The listing builds one solid part. Answer for the finished solid, in the listing's coordinates (mm). Face numbers are marked on the shaded views. A direction names the side the tool comes from. Round coordinates to 2 decimals unless told otherwise and drop trailing zeros. Loops run counter-clockwise (first coordinate to the right, second up) from the corner with the lowest first, then second, coordinate; pieces in that order, holes last. Notation, with made-up numbers: M 1,-13 L 43,-13 A36 cw 43,26 Z; hole C 39.5,35.25 d2. An arc over 180 degrees is marked long. Put each result on its own line as item: value. Start each with the question number.
(1) Section A-A, the plane x = 18.5 is taken. Determine the outline of the cut face in (y, z), then the cut area to 3 significant figures.
(2) Determine the mould class of the marked faces 6, 7 and 8 for opening direction Y: released by +Y, released by -Y, zero draft, split by the parting line, or undercut.
(3) Section C-C, the plane y = -60 is taken. Determine the outline of the cut face in (x, z), then the cut area to 3 significant figures.
(4) Section D-D, the plane y = 11 is taken. Determine the outline of the cut face in (x, z).
(5) Flat-ended cylindrical pins translate along their axes: P1, Ø22, axis at y = -7, z = 12, coming from the -X side; P2, Ø6, axis at y = -37, z = 26.5, coming from the -X side; P3, Ø2, axis at x = 184.5, z = 16.5, coming from the +Y side; P4, Ø12, axis at x = 85.5, y = -54, coming from the +Z side. Find the tip coordinate at first contact, or state that the pin passes through.
(6) Which of the six approach directions +Z, -Z, +X, -X, +Y, -Y give full straight-line access (tool end or side, diameter ignored) to the marked faces 1, 2, 3, 4 and 5?
(7) Straight lines are drawn through the part: line 1 (Y direction, x = 148, z = 12); line 2 (X direction, y = 34.5, z = 11); line 3 (Y direction, x = 180.5, z = 21). For each, find the intervals that lie inside material, in ascending order.
(8) Section B-B, the plane y = 36.5 is taken. Determine the outline of the cut face in (x, z), then the cut area to 3 significant figures.
```python
from build123d import *

# Parameters (mm, degrees)
BOSS_EXTRU_1_DEPTH      = 235
ESQUISSE2_R             = 28.575
ENL_V_MAT_EXTRU_1_DEPTH = 235
ESQUISSE3_R             = 44.45
ENL_V_MAT_EXTRU_2_DEPTH = 78
ESQUISSE4_W             = 33
ESQUISSE4_H             = 61.631350579
ENL_V_MAT_EXTRU_3_DEPTH = 19
ENL_V_MAT_EXTRU_4_DEPTH = 13
BOSS_EXTRU_2_START      = -33
BOSS_EXTRU_2_DEPTH      = 33


with BuildPart() as part:
    # Esquisse1 → Boss.-Extru.1 (new body)
    with BuildSketch(Plane(origin=(0, 0, 0), x_dir=(0, 0, -1), z_dir=(1, 0, 0))):
        with BuildLine():
            Line((0, 0), (0, 86))
            ThreePointArc((0, 86), (-60.811183182, 60.811183182), (-86, 0))
            Line((-86, 0), (-86, -43.853430349))
            Line((-86, -43.853430349), (-13, -86))
            Line((-13, -86), (0, -86))
            Line((0, -86), (0, 0))
        make_face()
    extrude(amount=BOSS_EXTRU_1_DEPTH)

    # Esquisse2 → Enlèv. mat.-Extru.1 (cut)
    with BuildSketch(Plane(origin=(0, 0, 0), x_dir=(0, 0, -1), z_dir=(1, 0, 0))):
        Circle(ESQUISSE2_R)
    extrude(amount=ENL_V_MAT_EXTRU_1_DEPTH, mode=Mode.SUBTRACT)

    # Esquisse3 → Enlèv. mat.-Extru.2 (cut)
    with BuildSketch(Plane(origin=(0, 0, 0), x_dir=(0, 0, -1), z_dir=(1, 0, 0))):
        Circle(ESQUISSE3_R)
    extrude(amount=ENL_V_MAT_EXTRU_2_DEPTH, mode=Mode.SUBTRACT)

    # Esquisse4 → Enlèv. mat.-Extru.3 (cut)
    with BuildSketch(Plane.XY):
        with Locations((180.5, 55.184324711)):
            Rectangle(ESQUISSE4_W, ESQUISSE4_H)
    extrude(amount=ENL_V_MAT_EXTRU_3_DEPTH, mode=Mode.SUBTRACT)

    # Esquisse5 → Enlèv. mat.-Extru.4 (cut)
    with BuildSketch(Plane.XY):
        with BuildLine():
            ThreePointArc((125, -71), (114, -60), (125, -49))
            Line((125, -49), (235, -49))
            Line((235, -49), (235, -71))
            Line((235, -71), (125, -71))
        make_face()
    extrude(amount=ENL_V_MAT_EXTRU_4_DEPTH, mode=Mode.SUBTRACT)

    # Esquisse6 → Boss.-Extru.2 (add)
    with BuildSketch(Plane(origin=(0, 0, 0), x_dir=(0, 0, -1), z_dir=(1, 0, 0)).offset(BOSS_EXTRU_2_START)):
        with BuildLine():
            Line((-65.430668922, -0.909705656), (-40.188548434, 31.398735242))
            Line((-40.188548434, 31.398735242), (-14.946427946, 63.707176139))
            Line((-14.946427946, 63.707176139), (-34.329616239, 78.850982549))
            ThreePointArc((-34.329616239, 78.850982549), (-67.683027015, 53.056647596), (-84.767274524, 14.508934135))
            Line((-84.767274524, 14.508934135), (-65.430668922, -0.909705656))
        make_face()
    extrude(amount=BOSS_EXTRU_2_DEPTH)


solid = part.part
```
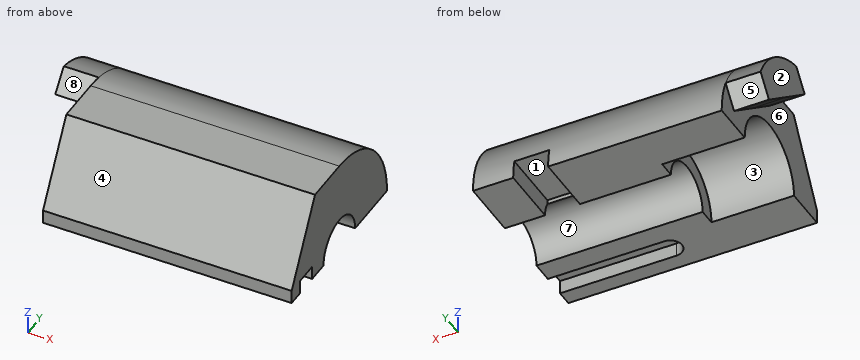
Recorded:
1. outline: M -86,0 L -44.45,0 A44.45 cw 44.45,0 L 86,0 A86 ccw 0,86 L -43.85,86 L -86,13 Z
1. area: 8,560 mm²
2. face 6: zero draft
2. face 7: undercut
2. face 8: released by -Y
3. outline: M 0,0 L 114,0 L 114,13 L 235,13 L 235,58.03 L 0,58.03 Z
3. area: 12,100 mm²
4. outline: M -33,56.13 L 0,56.13 L 0,43.07 L 78,43.07 L 78,26.37 L 235,26.37 L 235,85.29 L 0,85.29 L 0,80.37 L -33,80.37 Z
5. P1: passes through
5. P2: stops at x = 0
5. P3: stops at y = 24.37
5. P4: stops at z = 78.82
6. face 1: -Z, +Y
6. face 2: +Z, -Z, -X, +Y, -Y
6. face 3: -Z, -X
6. face 4: +Z, +X, -X, -Y
6. face 5: -Z, -X, +Y
7. line 1: y = -86 to -71, -49 to -25.93, 25.93 to 85.16
7. line 2: x = 78 to 164, 197 to 235
7. line 3: y = -81.38 to -19.38, 19.38 to 83.4
8. outline: M -33,36.2 L 0,36.2 L 0,25.37 L 78,25.37 L 78,0 L 164,0 L 164,19 L 197,19 L 197,0 L 235,0 L 235,77.87 L -33,77.87 Z
8. area: 17,100 mm²
